Answer from the drawing. Dimensions are ordinates in mm from the lowest x, y and z of the part. Give positions to 0.01 mm unless a question says otherwise; leave off trailing zeros. Write each loop counter-clockwise with the first axis right and the second up, starting at its lowest first coordinate (ties: lowest second). Pieces come first, ordered by that corner, then holes.
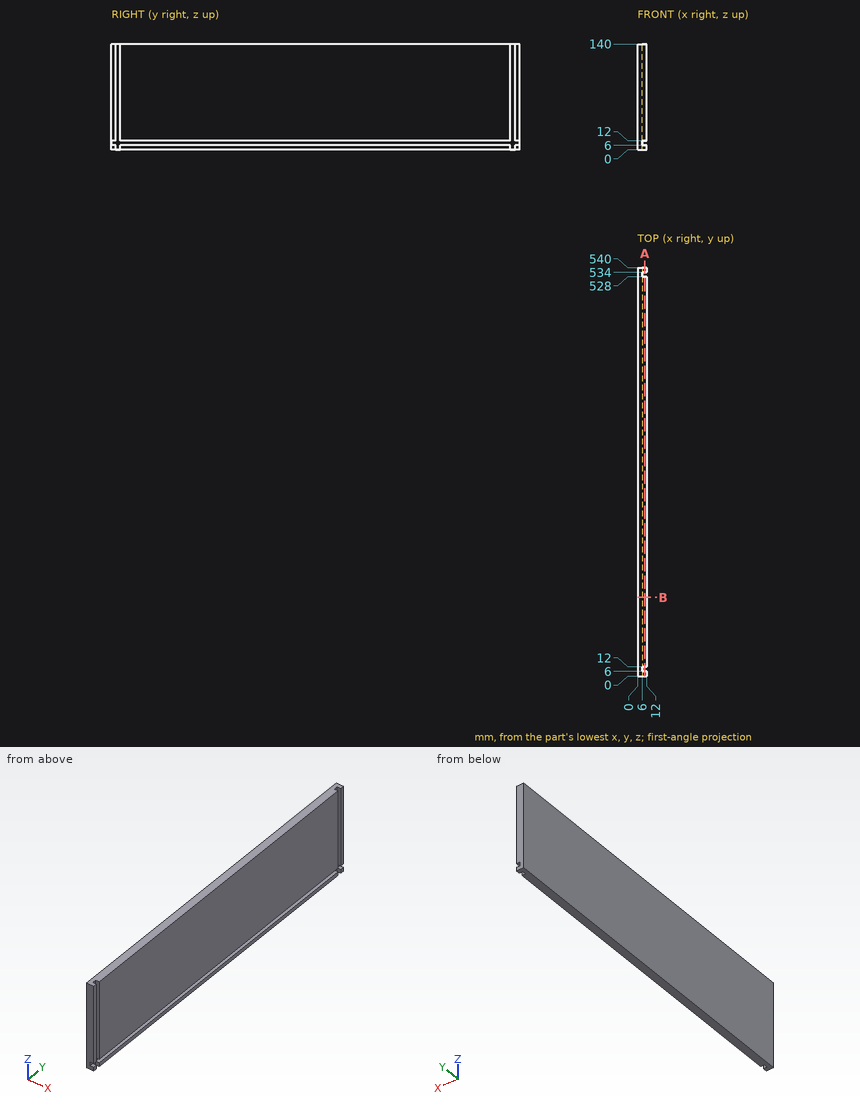
Item 1: Section B-B (y = 104) is taken. Write down the section's boundary in (x, z), and give its area (3 significant figures).
Result set:
outline: (0, 0) - (12, 0) - (12, 6) - (6, 6) - (6, 12) - (12, 12) - (12, 140) - (0, 140) - close
area: 1,640 mm2
Item 2: Section A-A (x = 9.75) is taken. Write down the section's boundary in (y, z).
Result set:
outline: (0, 0) - (6, 0) - (6, 6) - (0, 6) - close; (0, 12) - (6, 12) - (6, 140) - (0, 140) - close; (12, 0) - (528, 0) - (528, 6) - (12, 6) - close; (12, 12) - (528, 12) - (528, 140) - (12, 140) - close; (534, 0) - (540, 0) - (540, 6) - (534, 6) - close; (534, 12) - (540, 12) - (540, 140) - (534, 140) - close
Item 3: Find the intervals of material crossed by line 1 along Y through (x, z) = (6.5, 16.5); line 2 along Z through (x, y) = (9.25, 287); line 3 along X through (y, z) = (178, 9), in increasing order.
Result set:
line 1: y = 0 to 6, 12 to 528, 534 to 540
line 2: z = 0 to 6, 12 to 140
line 3: x = 0 to 6
